Here's how the part is built. I have some questions about the finished solid (model axes, mm). A direction names the side the tool comes from. Round coordinates to 2 decimals unless told otherwise and drop trailing zeros. Write each loop counter-clockwise with the first axis right and the second up, starting at its lowest first coordinate (ties: lowest second). Pieces come first, ordered by that corner, then holes. Notation, with made-up numbers: (-19.75, -5) - (5.25, -5) arc R10 cw to (5.25, 2) - close; hole circle Ø9 at (2, -38). An arc over 180 degrees is marked (long way). One line per item, written item: value. Start each with the question number.
Item 1: Imagine slicing it at B-B, the plane y = 26. Please give me the cut outline in (x, z).
Item 2: Thinking about a two-plate mould opening in X: for faces 1 (the face through (11.756, 2.394, 6.035)), 2 (the face through (13.8, 33, 3.5)), 3 (the face through (15.54, 33.84, 1.73)), which applies, released by +X, released by -X, zero draft, split by the parting line, or undercut?
Item 3: If I drill on line 1 (Y direction, x = 15, z = 10.1); line 2 (X direction, y = 3, z = 2.1); line 3 (X direction, y = 9, z = 6), over which ranges is the centre line in solid material (lowest first)?
Item 4: Imagine slicing it at C-C, the plane x = 14.5. Count the separate pieces of the cut face and the enclosed holes in it, then the cut area to 3 significant figures.
Item 5: For faces 4 (the face through (6.147, 6.471, 6.084)), 5 (the face through (0.301, 0.285, 6.084)), 6 (the face through (12.04, 0.47, 6.04)), 7 (the face through (6.466, 28.201, 5.916)), which set-ups out of +Z, -Z, +X, -X, +Y, -Y let a thin tool reach every point of the face, with its end or its side?
Item 6: Imagine slicing it at A-A, the plane z = 10. Please give me the cut outline in (x, y), then the cut area to 3 significant figures.
Item 7: Imagine slicing it at D-D, the plane y = 5.5. Please give me the cut outline in (x, z), then the cut area to 3 significant figures.
Item 8: For P1, Ø3, axis at x = 6.5, y = 20, coming from the +Z side; P2, Ø1.2, axis at x = 15, y = 33, coming from the -Z side; P3, Ø2, axis at y = 30, z = 3.5, coming from the +X side, each with a flat end and sliding along its axis, tell me the tip position at first contact or that it passes through.
```python
from build123d import *

# Parameters (mm, degrees)
SKETCH1_R               = 1
BOSS_EXTRUDE1_DEPTH     = 12
SKETCH2_R               = 3.3
CUT_EXTRUDE1_DEPTH      = 2.5
CUT_EXTRUDE1_DEPTH_BACK = 2.5
FILLET1_R               = 1
FILLET2_R               = 1
FILLET3_R               = 1
FILLET4_R               = 1


with BuildPart() as part:
    # Sketch1 → Boss-Extrude1 (new body)
    with BuildSketch(Plane.XY):
        with BuildLine():
            Line((0, 0), (15, 0))
            ThreePointArc((15, 0), (17.189317787, 5.051069873), (12.006370829, 3.19540825))
            Line((12.006370829, 3.19540825), (6, 6.391648207))
            Line((6, 6.391648207), (6, 19.92058514))
            Line((6, 19.92058514), (12.003141677, 33.137259573))
            ThreePointArc((12.003141677, 33.137259573), (17.072223598, 30.830693807), (15, 36))
            Line((15, 36), (0, 36))
            Line((0, 36), (0, 0))
        make_face()
        with Locations((15, 33)):
            Circle(SKETCH1_R, mode=Mode.SUBTRACT)
        with Locations((15, 3)):
            Circle(SKETCH1_R, mode=Mode.SUBTRACT)
        Polygon((8.708182188, 33.137259573), (3, 33.137259573), (3, 20.569975699), align=None, mode=Mode.SUBTRACT)
    extrude(amount=BOSS_EXTRUDE1_DEPTH)

    # Sketch2 → Cut-Extrude1 (cut, two sides)
    with BuildSketch(Plane.XY.offset(6)) as cut_extrude1_sk:
        with Locations((15, 33)):
            Circle(SKETCH2_R)
        with Locations((15, 3)):
            Circle(SKETCH2_R)
    extrude(amount=CUT_EXTRUDE1_DEPTH, mode=Mode.SUBTRACT)
    extrude(cut_extrude1_sk.sketch, amount=-CUT_EXTRUDE1_DEPTH_BACK, mode=Mode.SUBTRACT)

    # Fillet1
    fillet1_edges = [part.edges().sort_by_distance(p)[0] for p in [
        (0, 36, 6),
        (0, 0, 6),
    ]]
    fillet(fillet1_edges, radius=FILLET1_R)

    # Fillet2
    fillet2_edges = [part.edges().sort_by_distance(p)[0] for p in [
        (6, 19.92058514, 6),
        (6, 6.391648207, 6),
    ]]
    fillet(fillet2_edges, radius=FILLET2_R)

    # Fillet3
    fillet3_edges = [part.edges().sort_by_distance(p)[0] for p in [
        (13.625227292, 36, 6),
        (13.625227292, 0, 6),
    ]]
    fillet(fillet3_edges, radius=FILLET3_R)

    # Fillet4
    fillet4_edges = [part.edges().sort_by_distance(p)[0] for p in [
        (3, 20.569975699, 6),
        (8.708182188, 33.137259573, 6),
        (3, 33.137259573, 6),
    ]]
    fillet(fillet4_edges, radius=FILLET4_R)


solid = part.part
```
Values follow:
1. outline: (0, 0) - (3, 0) - (3, 12) - (0, 12) - close; (5.47, 0) - (8.76, 0) - (8.76, 12) - (5.47, 12) - close
2. face 1: released by +X
2. face 2: zero draft
2. face 3: undercut
3. line 1: y = 0 to 2, 4 to 6, 30 to 32, 34 to 36
3. line 2: x = 0 to 14, 16 to 18
3. line 3: x = 0 to 6
4. separate pieces: 8
4. enclosed holes: 0
4. area: 59.2 mm^2
5. face 4: +Z, -Z, +X
5. face 5: +Z, -Z, -X, -Y
5. face 6: +X
5. face 7: +Z, -Z
6. outline: (0, 1) arc R1 ccw to (1, 0) - (15, 0) arc R3 ccw (long way) to (12.01, 3.2) - (6.53, 6.11) arc R1 cw to (6, 6.99) - (6, 19.7) arc R1 cw to (6.09, 20.12) - (12, 33.14) arc R3 ccw (long way) to (15, 36) - (1, 36) arc R1 ccw to (0, 35) - close; hole (3, 25.19) arc R1 ccw to (4.91, 24.78) - (8.07, 31.72) arc R1 ccw to (7.16, 33.14) - (4, 33.14) arc R1 ccw to (3, 32.14) - close; hole circle Ø2 at (15, 3); hole circle Ø2 at (15, 33)
6. area: 324 mm^2
7. outline: (0, 0) - (7.68, 0) - (7.68, 12) - (0, 12) - close; (13.34, 0) - (16.66, 0) - (16.66, 3.5) - (13.34, 3.5) - close; (13.34, 8.5) - (16.66, 8.5) - (16.66, 12) - (13.34, 12) - close
7. area: 115 mm^2
8. P1: stops at z = 12
8. P2: passes through
8. P3: stops at x = 17.24
